The model under review builds one solid part; all positions refer to its coordinate system, in mm. A direction names the side the tool comes from. Coordinates: 2 decimals unless noted, no trailing zeros. Write each loop counter-clockwise with the first axis right and the second up, starting at its lowest first coordinate (ties: lowest second). Pieces come first, ordered by that corner, then holes. Notation, with made-up numbers: (84, 66) - (134, 66) arc R18 ccw to (134, 94) - close; hole circle Ø5 at (14, -6). An arc over 180 degrees is marked (long way). Put each result on its own line as item: value.
from build123d import *

# Parameters (mm, degrees)
EXTRU_MINCE1_DEPTH      = 4
CONG_1_R                = 1
CONG_2_R                = 3
ESQUISSE2_R             = 1.5
ENL_V_MAT_EXTRU_1_DEPTH = 36.156791793


with BuildPart() as part:
    # Esquisse1 → Extru.-Mince1 (new, symmetric)
    with BuildSketch(Plane(origin=(0, 0, 0), x_dir=(1, 0, 0), z_dir=(0, 1, 0))):
        with BuildLine():
            Line((-34, 0), (-3.069307952, 0))
            Line((-3.069307952, 0), (-3.863703305, 2.96472382))
            ThreePointArc((-3.863703305, 2.96472382), (0, 8), (3.863703305, 2.96472382))
            Line((3.863703305, 2.96472382), (3.069307952, 0))
            Line((3.069307952, 0), (34, 0))
            Line((34, 0), (34, 2))
            Line((34, 2), (5.675758698, 2))
            Line((5.675758698, 2), (5.795554958, 2.447085729))
            ThreePointArc((5.795554958, 2.447085729), (0, 10), (-5.795554958, 2.447085729))
            Line((-5.795554958, 2.447085729), (-5.675758698, 2))
            Line((-5.675758698, 2), (-34, 2))
            Line((-34, 2), (-34, 0))
        make_face()
    extrude(amount=EXTRU_MINCE1_DEPTH, both=True)

    # Congé1
    cong_1_edges = [part.edges().sort_by_distance(p)[0] for p in [
        (3.069307952, 0, 0),
        (-3.069307952, 0, 0),
    ]]
    fillet(cong_1_edges, radius=CONG_1_R)

    # Congé2
    cong_2_edges = [part.edges().sort_by_distance(p)[0] for p in [
        (34, -4, -1),
        (34, 4, -1),
        (5.675758698, 0, -2),
        (-34, -4, -1),
        (-34, 4, -1),
        (-5.675758698, 0, -2),
    ]]
    fillet(cong_2_edges, radius=CONG_2_R)

    # Esquisse2 → Enlèv. mat.-Extru.1 (cut, through all)
    with BuildSketch(Plane(origin=(0, 0, -2), x_dir=(-1, 0, 0), z_dir=(0, 0, -1))):
        with Locations((-30, 0)):
            Circle(ESQUISSE2_R)
        with Locations(Location((30, 0, 0), (0, 0, 180))):
            Circle(ESQUISSE2_R)
    extrude(amount=-ENL_V_MAT_EXTRU_1_DEPTH, mode=Mode.SUBTRACT)


solid = part.part
1. Consider section D-D on x = 0. State the section outline as (y, z) points.
Determined:
outline: (-4, -10) - (4, -10) - (4, -8) - (-4, -8) - close
2. For pin 1 Ø3.5 at (x, y) = (-30, 0) entering from -Z; pin 2 Ø4 at (y, z) = (-1.5, -2.5) entering from -X; pin 3 Ø2 at (y, z) = (-3, -2.5) entering from -X; pin 4 Ø2.5 at (x, y) = (30, 0) entering from -Z, all flat-tipped, find the tip position at first contact; note any pin that passes through.
Determined:
pin 1: stops at z = -2
pin 2: stops at x = -34
pin 3: stops at x = -33.78
pin 4: passes through
3. The part is to be moulded in two halves that separate along Y. For faces 1 (the flat face through (-5, 4, -3)), 2 (the cylindrical face through (-31.5, -0.07, -1.01)), 3 (the flat face through (-5, -4, -3)), 4 (the cylindrical face through (31.5, 0.07, -1.01)), say which applies: +Y half, -Y half, draft (parallel to the pull), parting line (faces both ways), or undercut.
Determined:
face 1: +Y half
face 2: undercut
face 3: -Y half
face 4: undercut
4. To check wall thickness, follow probe 1 along Y at (x, z) = (-30, -0.45); probe 2 along Z at (x, y) = (-16.5, -3.25); probe 3 along X at (y, z) = (3.75, -5.5). State the ranges of each line that lie inside material, in increasing order.
Determined:
probe 1: y = -4 to -1.5, 1.5 to 4
probe 2: z = -2 to 0
probe 3: x = -5.81 to -3.71, 3.71 to 5.81
5. Consider section A-A on x = -30. State the section outline as (y, z) points.
Determined:
outline: (-4, -2) - (-1.5, -2) - (-1.5, 0) - (-4, 0) - close; (1.5, -2) - (4, -2) - (4, 0) - (1.5, 0) - close
6. Machinability: for faces 5 (the flat face through (-3.63, 0.06, -2.1)), 6 (the flat face through (-21, 0, -2)), 7 (the flat face through (22, 0, -2)), 8 (the cylindrical face through (-33.1, -3.14, -0.99)), which of the approach directions +Z, -Z, +X, -X, +Y, -Y give a long, thin tool a straight path to every point of the face, cutting with its end or side? Answer none if there is none.
Determined:
face 5: +Y, -Y
face 6: -Z, -X, +Y, -Y
face 7: -Z, +X, +Y, -Y
face 8: +Z, -Z, -X, -Y
7. Consider section C-C on y = 0. Give the number of separate pieces and of enclosed holes in the cut face, plus the area to 3 significant figures.
Determined:
separate pieces: 3
enclosed holes: 0
area: 153 mm^2
8. Consider section B-B on z = -6.25. State the section outline as (x, y) points.
Determined:
outline: (-5.56, -4) - (-3.31, -4) - (-3.31, 4) - (-5.56, 4) - close; (3.31, -4) - (5.56, -4) - (5.56, 4) - (3.31, 4) - close
